from build123d import *

# Parameters (mm, degrees)
SKETCH1_W             = 100
SKETCH1_H             = 60
BOSS_EXTRUDE1_DEPTH   = 10
CUT_EXTRUDE1_REACH    = 12
SKETCH2_R             = 3
SKETCH2_R_2           = 4
SKETCH2_R_3           = 4.75
CUT_EXTRUDE2_DEPTH    = 3
M4_TAPPED_HOLE1_D     = 3.3
M4_TAPPED_HOLE1_DEPTH = 12
M4_TAPPED_HOLE1_TIP   = 0.991420021
M4_TAPPED_HOLE2_D     = 3.3
M4_TAPPED_HOLE2_DEPTH = 12
M4_TAPPED_HOLE2_TIP   = 0.991420021
M4_TAPPED_HOLE3_D     = 3.3
M4_TAPPED_HOLE3_DEPTH = 12
M4_TAPPED_HOLE3_TIP   = 0.991420021
M4_TAPPED_HOLE4_D     = 3.3
M4_TAPPED_HOLE4_DEPTH = 12
M4_TAPPED_HOLE4_TIP   = 0.991420021


with BuildPart() as part:
    # Sketch1 → Boss-Extrude1 (new body)
    with BuildSketch(Plane(origin=(0, 0, 0), x_dir=(1, 0, 0), z_dir=(0, 1, 0))):
        Rectangle(SKETCH1_W, SKETCH1_H)
    extrude(amount=BOSS_EXTRUDE1_DEPTH)

    # Sketch2 → Cut-Extrude1 (cut, up to next)
    with BuildSketch(Plane(origin=(0, 10, 0), x_dir=(1, 0, 0), z_dir=(0, 1, 0)), mode=Mode.PRIVATE) as cut_extrude1_sk1:
        with Locations((-40, 20)):
            Circle(SKETCH2_R)
    cut_extrude1_tool1 = extrude(cut_extrude1_sk1.sketch, amount=-CUT_EXTRUDE1_REACH, mode=Mode.PRIVATE) & part.part
    add(cut_extrude1_tool1.solids().sort_by_distance((-40, 10, -20))[0], mode=Mode.SUBTRACT)
    # Sketch2 → Cut-Extrude1 (cut, up to next)
    with BuildSketch(Plane(origin=(0, 10, 0), x_dir=(1, 0, 0), z_dir=(0, 1, 0)), mode=Mode.PRIVATE) as cut_extrude1_sk2:
        with Locations((-27, 20)):
            Circle(SKETCH2_R_2)
    cut_extrude1_tool2 = extrude(cut_extrude1_sk2.sketch, amount=-CUT_EXTRUDE1_REACH, mode=Mode.PRIVATE) & part.part
    add(cut_extrude1_tool2.solids().sort_by_distance((-27, 10, -20))[0], mode=Mode.SUBTRACT)
    # Sketch2 → Cut-Extrude1 (cut, up to next)
    with BuildSketch(Plane(origin=(0, 10, 0), x_dir=(1, 0, 0), z_dir=(0, 1, 0)), mode=Mode.PRIVATE) as cut_extrude1_sk3:
        with Locations((-2, 20)):
            Circle(SKETCH2_R_2)
    cut_extrude1_tool3 = extrude(cut_extrude1_sk3.sketch, amount=-CUT_EXTRUDE1_REACH, mode=Mode.PRIVATE) & part.part
    add(cut_extrude1_tool3.solids().sort_by_distance((-2, 10, -20))[0], mode=Mode.SUBTRACT)
    # Sketch2 → Cut-Extrude1 (cut, up to next)
    with BuildSketch(Plane(origin=(0, 10, 0), x_dir=(1, 0, 0), z_dir=(0, 1, 0)), mode=Mode.PRIVATE) as cut_extrude1_sk4:
        with Locations((23, 20)):
            Circle(SKETCH2_R_2)
    cut_extrude1_tool4 = extrude(cut_extrude1_sk4.sketch, amount=-CUT_EXTRUDE1_REACH, mode=Mode.PRIVATE) & part.part
    add(cut_extrude1_tool4.solids().sort_by_distance((23, 10, -20))[0], mode=Mode.SUBTRACT)
    # Sketch2 → Cut-Extrude1 (cut, up to next)
    with BuildSketch(Plane(origin=(0, 10, 0), x_dir=(1, 0, 0), z_dir=(0, 1, 0)), mode=Mode.PRIVATE) as cut_extrude1_sk5:
        with Locations((40, 20)):
            Circle(SKETCH2_R_3)
    cut_extrude1_tool5 = extrude(cut_extrude1_sk5.sketch, amount=-CUT_EXTRUDE1_REACH, mode=Mode.PRIVATE) & part.part
    add(cut_extrude1_tool5.solids().sort_by_distance((40, 10, -20))[0], mode=Mode.SUBTRACT)
    # Sketch2 → Cut-Extrude1 (cut, up to next)
    with BuildSketch(Plane(origin=(0, 10, 0), x_dir=(1, 0, 0), z_dir=(0, 1, 0)), mode=Mode.PRIVATE) as cut_extrude1_sk6:
        with Locations((-40, 7)):
            Circle(SKETCH2_R_2)
    cut_extrude1_tool6 = extrude(cut_extrude1_sk6.sketch, amount=-CUT_EXTRUDE1_REACH, mode=Mode.PRIVATE) & part.part
    add(cut_extrude1_tool6.solids().sort_by_distance((-40, 10, -7))[0], mode=Mode.SUBTRACT)
    # Sketch2 → Cut-Extrude1 (cut, up to next)
    with BuildSketch(Plane(origin=(0, 10, 0), x_dir=(1, 0, 0), z_dir=(0, 1, 0)), mode=Mode.PRIVATE) as cut_extrude1_sk7:
        with Locations((-40, -5)):
            Circle(SKETCH2_R_2)
    cut_extrude1_tool7 = extrude(cut_extrude1_sk7.sketch, amount=-CUT_EXTRUDE1_REACH, mode=Mode.PRIVATE) & part.part
    add(cut_extrude1_tool7.solids().sort_by_distance((-40, 10, 5))[0], mode=Mode.SUBTRACT)
    # Sketch2 → Cut-Extrude1 (cut, up to next)
    with BuildSketch(Plane(origin=(0, 10, 0), x_dir=(1, 0, 0), z_dir=(0, 1, 0)), mode=Mode.PRIVATE) as cut_extrude1_sk8:
        with Locations((-40, -20)):
            Circle(SKETCH2_R_3)
    cut_extrude1_tool8 = extrude(cut_extrude1_sk8.sketch, amount=-CUT_EXTRUDE1_REACH, mode=Mode.PRIVATE) & part.part
    add(cut_extrude1_tool8.solids().sort_by_distance((-40, 10, 20))[0], mode=Mode.SUBTRACT)

    # Sketch3 → Cut-Extrude2 (cut)
    with BuildSketch(Plane(origin=(0, 10, 0), x_dir=(1, 0, 0), z_dir=(0, 1, 0))):
        with BuildLine():
            Line((-46, 8.5), (-34, 8.5))
            ThreePointArc((-34, 8.5), (-32.5, 7), (-34, 5.5))
            Line((-34, 5.5), (-46, 5.5))
            ThreePointArc((-46, 5.5), (-47.5, 7), (-46, 8.5))
        make_face()
        with BuildLine():
            Line((-46, -3.5), (-34, -3.5))
            ThreePointArc((-34, -3.5), (-32.5, -5), (-34, -6.5))
            Line((-34, -6.5), (-46, -6.5))
            ThreePointArc((-46, -6.5), (-47.5, -5), (-46, -3.5))
        make_face()
        with BuildLine():
            Line((-25.5, 26), (-25.5, 14))
            ThreePointArc((-25.5, 14), (-27, 12.5), (-28.5, 14))
            Line((-28.5, 14), (-28.5, 26))
            ThreePointArc((-28.5, 26), (-27, 27.5), (-25.5, 26))
        make_face()
        with BuildLine():
            Line((-0.5, 26), (-0.5, 14))
            ThreePointArc((-0.5, 14), (-2, 12.5), (-3.5, 14))
            Line((-3.5, 14), (-3.5, 26))
            ThreePointArc((-3.5, 26), (-2, 27.5), (-0.5, 26))
        make_face()
        with BuildLine():
            Line((24.5, 26), (24.5, 14))
            ThreePointArc((24.5, 14), (23, 12.5), (21.5, 14))
            Line((21.5, 14), (21.5, 26))
            ThreePointArc((21.5, 26), (23, 27.5), (24.5, 26))
        make_face()
    extrude(amount=-CUT_EXTRUDE2_DEPTH, mode=Mode.SUBTRACT)

    # M4 Tapped Hole1
    with Locations(Plane.ZY.offset(50)):
        with Locations((20, 6)):
            Hole(M4_TAPPED_HOLE1_D / 2, depth=M4_TAPPED_HOLE1_DEPTH)
            with Locations((0, 0, -(M4_TAPPED_HOLE1_DEPTH + M4_TAPPED_HOLE1_TIP / 2))):  # 118° drill point
                Cone(0, M4_TAPPED_HOLE1_D / 2, M4_TAPPED_HOLE1_TIP, mode=Mode.SUBTRACT)

    # M4 Tapped Hole2
    with Locations(Plane.XY.offset(30)):
        with Locations((-40, 6), (-25, 5), (5, 5), (35, 5)):
            Hole(M4_TAPPED_HOLE2_D / 2, depth=M4_TAPPED_HOLE2_DEPTH)
            with Locations((0, 0, -(M4_TAPPED_HOLE2_DEPTH + M4_TAPPED_HOLE2_TIP / 2))):  # 118° drill point
                Cone(0, M4_TAPPED_HOLE2_D / 2, M4_TAPPED_HOLE2_TIP, mode=Mode.SUBTRACT)

    # M4 Tapped Hole3
    with Locations(Plane(origin=(50, 0, 0), x_dir=(0, 0, -1), z_dir=(1, 0, 0))):
        with Locations((-15, 5), (5, 5), (20, 6)):
            Hole(M4_TAPPED_HOLE3_D / 2, depth=M4_TAPPED_HOLE3_DEPTH)
            with Locations((0, 0, -(M4_TAPPED_HOLE3_DEPTH + M4_TAPPED_HOLE3_TIP / 2))):  # 118° drill point
                Cone(0, M4_TAPPED_HOLE3_D / 2, M4_TAPPED_HOLE3_TIP, mode=Mode.SUBTRACT)

    # M4 Tapped Hole4
    with Locations(Plane(origin=(0, 0, -30), x_dir=(-1, 0, 0), z_dir=(0, 0, -1))):
        with Locations((-40, 6)):
            Hole(M4_TAPPED_HOLE4_D / 2, depth=M4_TAPPED_HOLE4_DEPTH)
            with Locations((0, 0, -(M4_TAPPED_HOLE4_DEPTH + M4_TAPPED_HOLE4_TIP / 2))):  # 118° drill point
                Cone(0, M4_TAPPED_HOLE4_D / 2, M4_TAPPED_HOLE4_TIP, mode=Mode.SUBTRACT)


solid = part.part
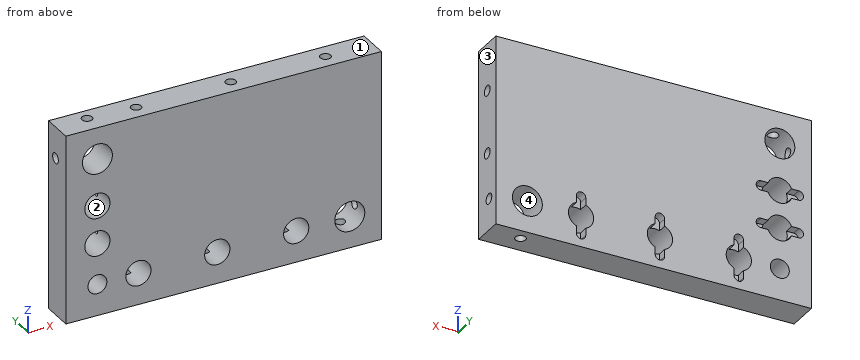
Here's how the part is built. I have some questions about the finished solid (model axes, mm). Face numbers are marked on the shaded views. Coordinates: 2 decimals unless noted, no trailing zeros. Write each loop counter-clockwise with the first axis right and the second up, starting at its lowest first coordinate (ties: lowest second). Pieces come first, ordered by that corner, then holes.
1) If we section it at A-A (x = 40): List the corners of the cut face in (y, z) for me.
Filled in:
outline: (0, -30) - (4.35, -30) - (4.35, -24.75) - (0, -24.75) - close; (0, -15.25) - (10, -15.25) - (10, 30) - (0, 30) - close; (7.65, -30) - (10, -30) - (10, -24.75) - (7.65, -24.75) - close; hole circle Ø3.3 at (5, -5); hole circle Ø3.3 at (5, 15)
2) If we section it at D-D (y = 2.25): Count the separate pieces of the cut face and the enclosed holes in it, plus the area to 3 significant figures.
Filled in:
separate pieces: 1
enclosed holes: 8
area: 5,580 mm2
3) If I drill on line 1 (X direction, y = 3.75, z = -20); line 2 (X direction, y = 6, z = -20); line 3 (Z direction, x = -40, y = 7), over which ranges is the centre line in solid material (lowest first)?
Filled in:
line 1: x = -50 to -43, -37 to -31, -23 to -6, 2 to 19, 27 to 35.25, 44.75 to 50
line 2: x = -50 to -43, -37 to -31, -23 to -6, 2 to 19, 27 to 35.25
line 3: z = -30 to -23, -17 to -11, -3 to 1, 9 to 15.25
4) If we section it at B-B (x = -2): List the corners of the cut face in (y, z) for me, plus the area to 3 significant figures.
Filled in:
outline: (0, -30) - (10, -30) - (10, -27.5) - (7, -27.5) - (7, -24) - (0, -24) - close; (0, -16) - (7, -16) - (7, -12.5) - (10, -12.5) - (10, 30) - (0, 30) - close
area: 499 mm2
5) I'm going to push flat-ended pins straight in: pin 1 (5.5 mm diameter, centred on x = 40, z = -20, fed in from -Y); pin 2 (2.5 mm diameter, centred on x = -2, z = -26, fed in from +Y); pin 3 (2.5 mm diameter, centred on x = 40, y = 6, fed in from -Z). Where does each tip first touch, or does it pass through?
Filled in:
pin 1: passes through
pin 2: stops at y = 7
pin 3: stops at z = -15.42
6) If we section it at C-C (z = -20): List the corners of the cut face in (x, y) for me.
Filled in:
outline: (-50, 0) - (-43, 0) - (-43, 10) - (-50, 10) - close; (-37, 0) - (-31, 0) - (-31, 10) - (-37, 10) - close; (-23, 0) - (-6, 0) - (-6, 10) - (-23, 10) - close; (2, 0) - (19, 0) - (19, 10) - (2, 10) - close; (27, 0) - (35.25, 0) - (35.25, 10) - (27, 10) - close; (44.75, 0) - (50, 0) - (50, 4.35) - (44.75, 4.35) - close; (44.75, 7.65) - (50, 7.65) - (50, 10) - (44.75, 10) - close
7) Thinking about a two-plate mould opening in X: for the marked faces 1, 2, 3 and 4, which applies, +X half, -X half, draft (parallel to the pull), parting line (faces both ways), or undercut?
Filled in:
face 1: draft
face 2: undercut
face 3: +X half
face 4: undercut
